Source: CAD feature listing. Evaluate the final solid. Frame: model axes, mm. Give positions to 0.01 mm unless a question says otherwise; leave off trailing zeros. Write each loop counter-clockwise with the first axis right and the second up, starting at its lowest first coordinate (ties: lowest second). Pieces come first, ordered by that corner, then holes.
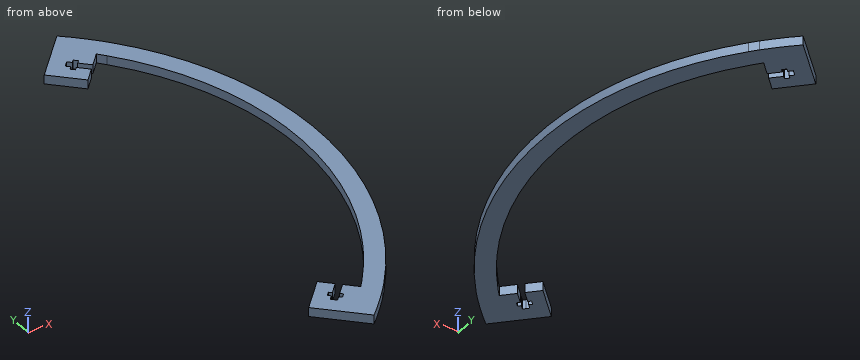
```python
from build123d import *

# Parameters (mm, degrees)
BOSS_EXTRUDE1_DEPTH = 6.35
BOSS_EXTRUDE3_START = -6.35
BOSS_EXTRUDE3_DEPTH = 6.35
CUT_EXTRUDE1_DEPTH  = 268.119964262


with BuildPart() as part:
    # Sketch1 → Boss-Extrude1 (new body)
    with BuildSketch(Plane.XY):
        with BuildLine():
            Line((143.360416784, 116.919323836), (134.344167558, 107.903074611))
            ThreePointArc((134.344167558, 107.903074611), (181.249035113, -21.950964887), (134.344167558, -151.805004385))
            Line((134.344167558, -151.805004385), (143.360416784, -160.82125361))
            ThreePointArc((143.360416784, -160.82125361), (193.949035113, -21.950964887), (143.360416784, 116.919323836))
        make_face()
    extrude(amount=BOSS_EXTRUDE1_DEPTH)

    # Sketch4 → Boss-Extrude3 (add)
    with BuildSketch(Plane.XY.offset(6.35).offset(BOSS_EXTRUDE3_START)):
        with BuildLine():
            Line((143.360416784, -160.82125361), (134.344167558, -151.805004385))
            ThreePointArc((134.344167558, -151.805004385), (132.290059148, -154.238328247), (130.198070847, -156.639163795))
            Line((130.198070847, -156.639163795), (139.193969877, -165.635062824))
            ThreePointArc((139.193969877, -165.635062824), (141.294938047, -163.24351662), (143.360416784, -160.82125361))
        make_face()
        with BuildLine():
            ThreePointArc((139.193969877, -165.635062824), (130.46291295, -174.865384883), (121.204013939, -183.56613137))
            Line((121.204013939, -183.56613137), (94.292689271, -156.654806703))
            Line((94.292689271, -156.654806703), (112.253201513, -138.694294461))
            Line((112.253201513, -138.694294461), (139.193969877, -165.635062824))
        make_face()
    boss_extrude3 = extrude(amount=BOSS_EXTRUDE3_DEPTH)

    # Sketch5 → Cut-Extrude1 (cut, through all)
    with BuildSketch(Plane.XY.offset(6.35)):
        Polygon((122.734319209, -149.175412156), (121.22563618, -147.666729128), (110.449328835, -158.443036473), (111.958011863, -159.951719502), (114.292878455, -157.61685291), (115.927285069, -159.251259524), (118.172349099, -157.006195494), (116.537942485, -155.37178888), align=None)
        Polygon((110.449328835, -158.443036473), (121.22563618, -147.666729128), (119.716953152, -146.1580461), (113.520576428, -152.354422823), (111.886169814, -150.720016209), (109.641105784, -152.965080239), (111.275512398, -154.599486854), (108.940645807, -156.934353445), align=None)
    cut_extrude1 = extrude(amount=-CUT_EXTRUDE1_DEPTH, mode=Mode.SUBTRACT)

    # Mirror2: Boss-Extrude3, Cut-Extrude1 across plane
    add(boss_extrude3.mirror(Plane.ZX.offset(-21.950964887)))
    add(cut_extrude1.mirror(Plane.ZX.offset(-21.950964887)), mode=Mode.SUBTRACT)


solid = part.part
```
1. Line query: probe 1 along Y at (x, z) = (113, 3.75); probe 2 along Y at (x, z) = (115, 4.75) (3 decimals); probe 3 along Y at (x, z) = (146.5, 0.5). Output: solid intervals per line, ascending.
2. Section query D-D (y = -8). Return loops of the section in (x, z), plus the area to 3 significant figures.
3. Section query C-C (y = 41). Return loops of the section in (x, z), plus the area to 3 significant figures.
4. Section query B-B (x = 102). Return loops of the section in (y, z).
5. Pin query (flat end, axial travel): P1, Ø2, axis at y = -70.5, z = 1.5, coming from the +X side; P2, Ø1, axis at y = -142.5, z = 5.5, coming from the -X side. Return the tip coordinate at first contact, or that it passes through.
6. Section query A-A (x = 173). Return loops of the section in (y, z).
The answers:
1. probe 1: y = -175.36 to -158.91, -151.83 to -139.44, 95.54 to 107.93, 115.01 to 131.46
1. probe 2: y = -177.362 to -158.324, -150.875 to -141.441, 97.539 to 106.973, 114.422 to 133.46
1. probe 3: y = -157 to -135.59, 91.69 to 113.09
2. outline: (180.77, 0) - (193.5, 0) - (193.5, 6.35) - (180.77, 6.35) - close
2. area: 80.8 mm2
3. outline: (171.25, 0) - (184.57, 0) - (184.57, 6.35) - (171.25, 6.35) - close
3. area: 84.6 mm2
4. outline: (-164.36, 0) - (-148.95, 0) - (-148.95, 6.35) - (-164.36, 6.35) - close; (105.05, 0) - (120.46, 0) - (120.46, 6.35) - (105.05, 6.35) - close
5. P1: stops at x = 188.65
5. P2: stops at x = 107.95
6. outline: (-114.72, 0) - (-79.26, 0) - (-79.26, 6.35) - (-114.72, 6.35) - close; (35.36, 0) - (70.82, 0) - (70.82, 6.35) - (35.36, 6.35) - close
